```python
from build123d import *

# Parameters (mm, degrees)
F0_W           = 30
F0_H           = 22
F1_DEPTH       = 3
F2_W           = 30
F2_H           = 5
F2_R           = 4
F3_DEPTH       = 10
F3_TAPER       = 8
F4_DEPTH       = 12
F6_D           = 5.6
F6_DEPTH       = 15
F6_CBORE_D     = 10
F6_CBORE_DEPTH = 2
F6_TIP         = 1.6824097333


with BuildPart() as f1:
    # F0 (on Top) → F1 (new body)
    with BuildSketch(Plane.XY):
        with Locations((0.4801530018, 11)):
            Rectangle(F0_W, F0_H)
    extrude(amount=F1_DEPTH)

    # F2 (on face) → F3 (join)
    with BuildSketch(Plane.XY.offset(3)):
        with Locations((0.4801530018, 2.5)):
            Rectangle(F2_W, F2_H)
        with Locations((0, 17.5365079194)):
            Circle(F2_R)
    extrude(amount=F3_DEPTH, taper=F3_TAPER)

    # F2 (on face) → F4 (join)
    with BuildSketch(Plane.XY.offset(3)):
        with Locations((0.4801530018, 2.5)):
            Rectangle(F2_W, F2_H)
    extrude(amount=F4_DEPTH)

    # F6
    with Locations(Plane(origin=(0, 5, 0), x_dir=(-1, 0, 0), z_dir=(0, 1, 0))):
        with Locations((-8.9809922501, 8.6309639737)):
            CounterBoreHole(F6_D / 2, F6_CBORE_D / 2, F6_CBORE_DEPTH, depth=F6_DEPTH)
            with Locations((0, 0, -(F6_DEPTH + F6_TIP / 2))):  # 118° drill point
                Cone(0, F6_D / 2, F6_TIP, mode=Mode.SUBTRACT)


solid = f1.part
```
The listing builds one solid part. Answer for the finished solid, in the listing's coordinates (mm). A direction names the side the tool comes from. Give positions to 0.01 mm unless a question says otherwise; leave off trailing zeros. Write each loop counter-clockwise with the first axis right and the second up, starting at its lowest first coordinate (ties: lowest second). Pieces come first, ordered by that corner, then holes. Notation, with made-up numbers: (59.25, 77) -> (86.25, 77) arc R23 ccw to (86.25, 110) -> close; hole circle Ø9 at (34, -16). An arc over 180 degrees is marked (long way). Write item = value, one per line. Start each with the question number.
1) Which of the six approach directions +Z, -Z, +X, -X, +Y, -Y give full straight-line access (tool end or side, diameter ignored) to faces 1 (the face through (-3, 5, 9)), 2 (the face through (0, 12, 3)), 3 (the face through (12.95, 4.01, 5.59)), 4 (the face through (0, 18, 13))?
2) The part is cut by section A-A, the plane z = 10. Determine the outline of the cut face in (x, y).
3) The part is cut by section C-C, the plane x = 9. Determine the outline of the cut face in (y, z), and give its area (3 significant figures).
4) The part is cut by section B-B, the plane x = -5.25. Determine the outline of the cut face in (y, z).
5) The part is cut by section D-D, the plane z = 12.25. Determine the outline of the cut face in (x, y), and give its area (3 significant figures).
6) Determine the mould class of faces 5 (the face through (0, 3, 15)), 6 (the face through (7, 3, 6)), 7 (the face through (0, 11, 0)) for opening direction Z: +Z half, -Z half, draft (parallel to the pull), parting line (faces both ways), or undercut.
7) Straight lines are drawn through the part: line 1 along Y through (x, z) = (11.25, 5.75); line 2 along X through (y, z) = (2, 8.5). For each, find the intervals that lie inside material, in ascending order.
8) Each of these flat-tipped pins is pushed along its axis until it touches: pin 1 (10 mm diameter, centred on x = -1.5, y = 15.5, fed in from +Z); pin 2 (2 mm diameter, centred on x = -3.5, y = 11, fed in from +Z); pin 3 (9 mm diameter, centred on x = 8.98, z = 8.63, fed in from +Y); pin 4 (3.5 mm diameter, centred on x = 8.98, z = 8.63, fed in from +Y) (3 decimals). Where does it stop, or does it pass through?
Solutions:
q1.face_1 = +Z, +X, -X
q1.face_2 = +Z
q1.face_3 = +Y
q1.face_4 = +Z, +X, -X, +Y
q2.outline = (-14.52, 0) -> (6.54, 0) -> (6.54, 3) -> (4.17, 3) -> (4.17, 5) -> (-14.52, 5) -> close; circle Ø6.03 at (0, 17.54); (11.42, 0) -> (15.48, 0) -> (15.48, 5) -> (13.79, 5) -> (13.79, 3) -> (11.42, 3) -> close
q3.outline = (0, 0) -> (22, 0) -> (22, 3) -> (5, 3) -> (5, 3.63) -> (3, 3.63) -> (3, 5.83) -> (0, 5.83) -> close; (0, 11.43) -> (3, 11.43) -> (3, 13.63) -> (5, 13.63) -> (5, 15) -> (0, 15) -> close
q3.area = 89.2 mm²
q4.outline = (0, 0) -> (22, 0) -> (22, 3) -> (5, 3) -> (5, 15) -> (0, 15) -> close
q5.outline = (-14.52, 0) -> (15.48, 0) -> (15.48, 5) -> (12.43, 5) -> (12.43, 3) -> (5.53, 3) -> (5.53, 5) -> (-14.52, 5) -> close; circle Ø5.4 at (0, 17.54)
q5.area = 159 mm²
q6.face_5 = +Z half
q6.face_6 = undercut
q6.face_7 = -Z half
q7.line_1 = 0 to 3
q7.line_2 = -14.52 to 6.18, 11.78 to 15.48
q8.pin_1 = 13
q8.pin_2 = 3
q8.pin_3 = 3
q8.pin_4 = through
